Source: CAD feature listing. Evaluate the final solid. Frame: model axes, mm. A direction names the side the tool comes from. Coordinates: 2 decimals unless noted, no trailing zeros. Order: outer loops, then holes, each group sorted by start corner. A loop starts at its lowest first (then second) coordinate and runs counter-clockwise, first axis right, second up. Notation, with made-up numbers: (80.5, -24.5) - (135.5, -24.5) arc R22 cw to (135.5, -16.5) - close; hole circle Ø5 at (-3, 35). An arc over 180 degrees is marked (long way). One line per question, with ' | ' between items. Start each with the question number.
(1) Section A-A (z = 332). Return the cut outline in (x, y), then the cut area to 3 significant figures.
(2) Contact query for flat-ended pins moving along their axis: P1, Ø7.5, axis at x = 186.5, y = -11.5, coming from the +Z side; P2, Ø1, axis at x = 257, z = 582.5, coming from the +Y side; P3, Ø1, axis at x = 648.5, z = 276.5, coming from the +Y side; P4, Ø8, axis at y = 127, z = 201, coming from the -X side. Output: stop coordinate, or through.
(3) Section D-D (y = 298). Return the cut outline in (x, z).
(4) Section B-B (x = 333.5). Return the cut outline in (y, z), then the cut area to 3 significant figures.
(5) Section C-C (z = 137). Return the cut outline in (x, y).
(6) Line query: line 1 along Y through (x, z) = (148, 661); line 2 along X through (y, z) = (92.5, 163); line 3 along Z through (x, y) = (85, 84). Output: solid intervals per line, ascending.
(7) Draft query along Y for faces 1 (the cylindrical face through (396.499, 337.313, 528.478)), 2 (the cylindrical face through (540.41, 518.921, 156.835)), 3 (the cylindrical face through (231.034, 155.903, 549.168)). Return one class per face: +Y half, -Y half, draft (parallel to the pull), parting line (faces both ways), or undercut.
(8) Access query for faces 4 (the flat face through (134.52, 100.89, 183.71)), 5 (the flat face through (400.62, 376.14, 236.75)), 6 (the cylindrical face through (277.117, 188.816, 183.741)). Directions: +Z, -Z, +X, -X, +Y, -Y. A direction counts if a zero-diameter tool reaches every point of the face in a straight line with its end or side. Return the directions, or none.
from build123d import *

# Parameters (mm, degrees)
BOSS_EXTRUDE1_DEPTH  = 152.4
CUT_EXTRUDE1_DEPTH   = 406.4
BOSS_EXTRUDE2_DEPTH  = 406.4
CUT_EXTRUDE3_DEPTH   = 508
BOSS_EXTRUDE3_DEPTH  = 25.4
BOSS_EXTRUDE4_DEPTH  = 25.4
BOSS_EXTRUDE5_DEPTH  = 12.7
BOSS_EXTRUDE6_DEPTH  = 12.7
CUT_EXTRUDE4_START   = -406.4
CUT_EXTRUDE4_DEPTH   = 406.4
FILLET1_R            = 25.4
SKETCH16_W           = 406.4
SKETCH16_H           = 431.79999999999995
BOSS_EXTRUDE8_DEPTH  = 5.08
CUT_EXTRUDE5_DEPTH   = 508
SKETCH20_W           = 25.39999999999924
SKETCH20_H           = 279.40000000000003
CUT_EXTRUDE6_DEPTH   = 508
BOSS_EXTRUDE9_DEPTH  = 40.64
SKETCH22_R           = 63.50000000000003
SKETCH22_R_2         = 63.49999999999997
BOSS_EXTRUDE10_DEPTH = 40.64
SKETCH23_R           = 38.1
CUT_EXTRUDE7_DEPTH   = 279.4
SKETCH24_W           = 279.4
SKETCH24_H           = 50.542616051246114
CUT_EXTRUDE8_DEPTH   = 182.88000000000048
SKETCH25_R           = 38.1
BOSS_EXTRUDE11_DEPTH = 279.4
BOSS_EXTRUDE12_DEPTH = 63.50000000000077
BOSS_EXTRUDE14_DEPTH = 63.50000000000077
SKETCH32_W           = 67.04968691962685
SKETCH32_H           = 63.49999999999994
SKETCH32_W_2         = 67.73333333333292
SKETCH32_H_2         = 63.49999999999997
BOSS_EXTRUDE15_DEPTH = 101.6
CUT_EXTRUDE9_DEPTH   = 25.4
SKETCH34_W           = 25.40000000000001
SKETCH34_H           = 101.6
CUT_EXTRUDE11_DEPTH  = 304.8
SKETCH36_R           = 12.7
BOSS_EXTRUDE16_DEPTH = 317.5


with BuildPart() as part:
    # Sketch1 → Boss-Extrude1 (new body)
    with BuildSketch(Plane(origin=(0, 0, 0), x_dir=(1, 0, 0), z_dir=(0, 1, 0))):
        Polygon((0, 0), (812.8, 0), (812.8000000000001, -711.1999999999999), (0, -711.1999999999999), align=None)
    extrude(amount=BOSS_EXTRUDE1_DEPTH)

    # Sketch2 → Cut-Extrude1 (cut)
    with BuildSketch(Plane(origin=(0, 0, 152.4), x_dir=(-1, 0, 0), z_dir=(0, 0, -1))):
        Polygon((0, 0), (-203.2, 152.4), (0, 152.4), align=None)
    extrude(amount=-CUT_EXTRUDE1_DEPTH, mode=Mode.SUBTRACT)

    # Sketch5 → Boss-Extrude2 (add)
    with BuildSketch(Plane.XY.offset(558.8)):
        Polygon((203.2, 152.4), (521.495119519974, 548.3194575791465), (554.1241709988542, 522.0876883607381), (256.91779556245336, 152.39999999999998), align=None)
    extrude(amount=-BOSS_EXTRUDE2_DEPTH)

    # Sketch6 → Cut-Extrude3 (cut)
    with BuildSketch(Plane(origin=(472.48898283734724, 587.7174054041558, 0), x_dir=(0.7793690109825708, -0.6265651959054618, 0), z_dir=(0.6265651959054618, 0.7793690109825708, 0))):
        Polygon((62.87924717566551, -203.2), (104.74523237533951, -203.2), (104.74523237533951, -508), (62.87924717566555, -508), align=None)
    extrude(amount=-CUT_EXTRUDE3_DEPTH, mode=Mode.SUBTRACT)

    # Sketch8 → Boss-Extrude3 (add)
    with BuildSketch(Plane(origin=(81.63518816150813, -65.62971704341768, 0), x_dir=(0, 0, -1), z_dir=(0.7793690109825717, -0.6265651959054606, 0))):
        Polygon((-558.8, 754.0938850817336), (-508, 754.0938850817336), (-508, 246.0938850817336), (-558.7999999999998, 246.0938850817336), align=None)
    extrude(amount=BOSS_EXTRUDE3_DEPTH)

    # Sketch9 → Boss-Extrude4 (add)
    with BuildSketch(Plane(origin=(81.63518816150813, -65.62971704341768, 0), x_dir=(0, 0, -1), z_dir=(0.7793690109825717, -0.6265651959054606, 0))):
        Polygon((-203.2, 754.0938850817341), (-152.39999999999998, 754.0938850817341), (-152.39999999999998, 246.09388508173413), (-203.19999999999993, 246.09388508173413), align=None)
    extrude(amount=BOSS_EXTRUDE4_DEPTH)

    # Sketch10 → Boss-Extrude5 (add)
    with BuildSketch(Plane.XY.offset(203.2)):
        Polygon((203.1999999999997, 152.40000000000092), (521.4951195199743, 548.319457579147), (573.920143877812, 506.1729323847398), (289.50826251979043, 152.39999999999992), (256.9177955624533, 152.39999999999986), (235.82905147888056, 126.16823078159206), align=None)
    extrude(amount=BOSS_EXTRUDE5_DEPTH)

    # Sketch11 → Boss-Extrude6 (add)
    with BuildSketch(Plane(origin=(0, 0, 508), x_dir=(-1, 0, 0), z_dir=(0, 0, -1))):
        Polygon((-573.9201438778116, 506.1729323847395), (-289.5082625197906, 152.40000000000015), (-256.91779556245325, 152.39999999999995), (-235.82905147888056, 126.16823078159206), (-203.1999999999997, 152.40000000000092), (-521.4951195199743, 548.319457579147), align=None)
    extrude(amount=BOSS_EXTRUDE6_DEPTH)

    # Sketch12 → Cut-Extrude4 (cut)
    with BuildSketch(Plane(origin=(0, 0, 152.39999999999975), x_dir=(-1, 0, 0), z_dir=(0, 0, -1)).offset(CUT_EXTRUDE4_START)):
        Polygon((-272.8899527583018, 152.4), (-543.4408043502763, 488.93153894227703), (-512.5781156253607, 513.7432601354462), (-222.08015203498906, 152.39999999999998), align=None)
    extrude(amount=CUT_EXTRUDE4_DEPTH, mode=Mode.SUBTRACT)

    # Fillet1
    fillet1_edges = [part.edges().sort_by_distance(p)[0] for p in [
        (547.7076316988932, 527.2461949819434, 215.89999999999998),
        (547.707631698893, 527.2461949819433, 495.3),
        (547.707631698893, 527.2461949819432, 152.39999999999998),
        (521.4951195199742, 548.3194575791467, 184.14999999999998),
        (547.7076316988928, 527.246194981943, 558.8),
        (521.4951195199742, 548.3194575791467, 527.05),
        (573.9201438778116, 506.17293238473945, 527.05),
        (573.920143877812, 506.17293238473985, 184.14999999999998),
    ]]
    fillet(fillet1_edges, radius=FILLET1_R)

    # Sketch16 → Boss-Extrude8 (add)
    with BuildSketch(Plane(origin=(101.43116104046555, -81.54447301941644, 0), x_dir=(0, 0, -1), z_dir=(0.7793690109825715, -0.6265651959054606, 0))):
        with Locations((-355.59999999999997, 512.7938850817336)):
            Rectangle(SKETCH16_W, SKETCH16_H)
    extrude(amount=BOSS_EXTRUDE8_DEPTH)

    # Sketch18 → Cut-Extrude5 (cut)
    with BuildSketch(Plane(origin=(154.19386331737303, 191.79794782500986, 0), x_dir=(0.7793690109825709, -0.6265651959054616, 0), z_dir=(0.6265651959054614, 0.7793690109825708, 0))):
        Polygon((62.8792471756653, -215.89999999999998), (4.163e-14, -215.89999999999998), (4.163e-14, -495.3), (62.8792471756653, -495.3), (104.74523237533926, -495.3), (130.1452323753393, -495.3), (130.14523237533894, -215.89999999999998), (104.74523237533926, -215.89999999999998), align=None)
    extrude(amount=-CUT_EXTRUDE5_DEPTH, mode=Mode.SUBTRACT)

    # Sketch20 → Cut-Extrude6 (cut)
    with BuildSketch(Plane(origin=(154.19386331737306, 191.79794782500986, 0), x_dir=(-0.7793690109825709, 0.6265651959054614, 0), z_dir=(-0.6265651959054614, -0.7793690109825709, 0))):
        with Locations((-117.44523237533932, -355.6)):
            Rectangle(SKETCH20_W, SKETCH20_H)
    extrude(amount=-CUT_EXTRUDE6_DEPTH, mode=Mode.SUBTRACT)

    # Sketch21 → Boss-Extrude9 (add)
    with BuildSketch(Plane(origin=(91.33693287972456, -73.42932864502501, 0), x_dir=(0, 0, 1), z_dir=(-0.7793690109825776, 0.6265651959054531, 0))):
        with BuildLine():
            Line((209.39759999999998, 562.2934659364746), (289.1018868532613, 546.366600042237))
            Line((289.1018868532613, 546.366600042237), (210.56545348218663, 525.4269956202154))
            ThreePointArc((210.56545348218663, 525.4269956202154), (185.1552700280405, 511.30785991563), (158.90239999999997, 523.7904170057728))
            Line((158.90239999999997, 523.7904170057728), (79.93520930816898, 543.0419414711238))
            Line((79.93520930816898, 543.0419414711238), (158.90239999999997, 562.2934659364746))
            ThreePointArc((158.90239999999997, 562.2934659364746), (184.14999999999998, 574.7919414711238), (209.39759999999998, 562.2934659364746))
        make_face()
        with BuildLine():
            Line((289.1018868532613, 292.366600042237), (210.56545348218663, 271.42699562021545))
            ThreePointArc((210.56545348218663, 271.42699562021545), (185.15527002804046, 257.30785991563005), (158.90239999999997, 269.7904170057729))
            Line((158.90239999999997, 269.7904170057729), (79.93520930816898, 289.0419414711237))
            Line((79.93520930816898, 289.0419414711237), (158.90239999999997, 308.29346593647455))
            ThreePointArc((158.90239999999997, 308.29346593647455), (184.14999999999998, 320.7919414711238), (209.39759999999998, 308.29346593647455))
            Line((209.39759999999998, 308.29346593647455), (289.1018868532613, 292.366600042237))
        make_face()
        with BuildLine():
            Line((632.0018868532613, 292.36660004223734), (553.4654534821866, 271.4269956202158))
            ThreePointArc((553.4654534821866, 271.4269956202158), (528.0552700280405, 257.3078599156303), (501.8024, 269.79041700577324))
            Line((501.8024, 269.79041700577324), (422.835209308169, 289.04194147112406))
            Line((422.835209308169, 289.04194147112406), (501.8024, 308.2934659364749))
            ThreePointArc((501.8024, 308.2934659364749), (527.0500000000001, 320.791941471124), (552.2976, 308.2934659364749))
            Line((552.2976, 308.2934659364749), (632.0018868532613, 292.36660004223734))
        make_face()
        with BuildLine():
            Line((501.8024, 523.7904170057732), (422.835209308169, 543.041941471124))
            Line((422.835209308169, 543.041941471124), (501.8024, 562.293465936475))
            ThreePointArc((501.8024, 562.293465936475), (527.0500000000001, 574.791941471124), (552.2976, 562.293465936475))
            Line((552.2976, 562.293465936475), (632.0018868532613, 546.3666000422373))
            Line((632.0018868532613, 546.3666000422373), (553.4654534821866, 525.4269956202157))
            ThreePointArc((553.4654534821866, 525.4269956202157), (528.0552700280405, 511.3078599156302), (501.8024, 523.7904170057732))
        make_face()
    extrude(amount=BOSS_EXTRUDE9_DEPTH)

    # Sketch22 → Boss-Extrude10 (add)
    with BuildSketch(Plane(origin=(91.33693287972456, -73.42932864502501, 0), x_dir=(0, 0, 1), z_dir=(-0.7793690109825776, 0.6265651959054531, 0))):
        with Locations((184.14999999999998, 670.4976110611291)):
            Circle(SKETCH22_R)
        with Locations((519.43, 670.4976110611292)):
            Circle(SKETCH22_R_2)
    extrude(amount=BOSS_EXTRUDE10_DEPTH)

    # Sketch23 → Cut-Extrude7 (cut)
    with BuildSketch(Plane.XY.offset(215.89999999999998)):
        with Locations((203.2, 12.700000000001378)):
            Circle(SKETCH23_R)
    extrude(amount=CUT_EXTRUDE7_DEPTH, mode=Mode.SUBTRACT)

    # Sketch24 → Cut-Extrude8 (cut)
    with BuildSketch(Plane.ZY):
        with Locations((355.59999999999997, 25.271308025623057)):
            Rectangle(SKETCH24_W, SKETCH24_H)
    extrude(amount=-CUT_EXTRUDE8_DEPTH, mode=Mode.SUBTRACT)

    # Sketch25 → Boss-Extrude11 (add)
    with BuildSketch(Plane.XY.offset(215.89999999999998)):
        with Locations((203.2, 12.700000000001378)):
            Circle(SKETCH25_R)
    extrude(amount=BOSS_EXTRUDE11_DEPTH)

    # Sketch26 → Boss-Extrude12 (add)
    with BuildSketch(Plane.XY.offset(215.89999999999998)):
        Polygon((0, 0), (-6.22e-15, 50.8), (67.73333333333265, 50.8), align=None)
    extrude(amount=-BOSS_EXTRUDE12_DEPTH)

    # Sketch30 → Boss-Extrude14 (add)
    with BuildSketch(Plane(origin=(0, 0, 495.3), x_dir=(-1, 0, 0), z_dir=(0, 0, -1))):
        Polygon((2.776e-14, -2.776e-14), (0, 50.79999999999997), (-67.73333333333278, 50.79999999999996), align=None)
    extrude(amount=-BOSS_EXTRUDE14_DEPTH)

    # Sketch32 → Boss-Extrude15 (add)
    with BuildSketch(Plane(origin=(5.2e-15, 50.79999999999997, 0), x_dir=(1, -1e-16, 0), z_dir=(1e-16, 1, 0))):
        with Locations((33.524843459813425, -527.05)):
            Rectangle(SKETCH32_W, SKETCH32_H)
        with Locations((33.86666666666645, -184.14999999999998)):
            Rectangle(SKETCH32_W_2, SKETCH32_H_2)
    extrude(amount=BOSS_EXTRUDE15_DEPTH)

    # Sketch33 → Cut-Extrude9 (cut)
    with BuildSketch(Plane.XY.offset(215.89999999999998)):
        Polygon((12.69999999999997, 134.2251095976107), (38.099999999999966, 134.2251095976107), (38.09999999999998, 32.625109597610695), (12.699999999999983, 32.625109597610695), align=None)
    extrude(amount=-CUT_EXTRUDE9_DEPTH, mode=Mode.SUBTRACT)

    # Sketch34 → Cut-Extrude11 (cut)
    with BuildSketch(Plane.XY.offset(215.89999999999998)):
        with Locations((25.399999999999977, 83.4251095976107)):
            Rectangle(SKETCH34_W, SKETCH34_H)
    extrude(amount=CUT_EXTRUDE11_DEPTH, mode=Mode.SUBTRACT)

    # Sketch36 → Boss-Extrude16 (add)
    with BuildSketch(Plane.XY.offset(190.49999999999997)):
        with Locations(Location((29.63333333333292, 108.82510959761069, 0), (0, 0, 311.810314896))):
            Circle(SKETCH36_R)
    extrude(amount=BOSS_EXTRUDE16_DEPTH)


solid = part.part
Response values:
1) outline: circle Ø25.4 at (29.63, 108.83); (207.62, 50.54) arc R38.1 ccw (long way) to (239.12, 0) - (812.8, 0) - (812.8, 152.4) - (296.03, 152.4) - (561.96, 483.19) - (558.01, 486.38) - close | area: 93,900 mm²
2) P1: stops at z = 495.3 | P2: stops at y = 181.63 | P3: stops at y = 152.4 | P4: stops at x = 0
3) outline: (320.25, 152.4) - (339.13, 152.4) - (339.13, 215.9) - (320.25, 215.9) - close; (320.25, 495.3) - (339.13, 495.3) - (339.13, 558.8) - (320.25, 558.8) - close; (389.94, 152.4) - (413.08, 152.4) - (413.08, 558.8) - (389.94, 558.8) - (389.94, 495.3) - (406.56, 495.3) - (406.56, 215.9) - (389.94, 215.9) - close
4) outline: (0, 0) - (152.4, 0) - (152.4, 711.2) - (0, 711.2) - close; (199.01, 152.4) - (227.79, 152.4) - (227.79, 215.9) - (207.12, 215.9) - (207.12, 495.3) - (227.79, 495.3) - (227.79, 558.8) - (199.01, 558.8) - close; (290.99, 152.4) - (314.48, 152.4) - (314.48, 215.9) - (290.99, 215.9) - close; (290.99, 495.3) - (314.48, 495.3) - (314.48, 558.8) - (290.99, 558.8) - close | area: 117,000 mm²
5) outline: (0, 0) - (812.8, 0) - (812.8, 152.4) - (272.89, 152.4) - (281.16, 162.68) - (249.48, 188.15) - (232.05, 166.46) - (249.54, 152.4) - (0, 152.4) - close; (391.2, 364.42) - (422.87, 338.96) - (440.3, 360.64) - (408.63, 386.11) - close; (453.12, 441.45) - (484.8, 415.99) - (538.1, 482.29) - (506.42, 507.75) - close
6) line 1: y = 0 to 152.4 | line 2: x = 0 to 67.73, 123.33 to 812.8 | line 3: z = 0 to 152.4, 558.8 to 711.2
7) face 1: undercut | face 2: +Y half | face 3: undercut
8) face 4: +Y | face 5: -X, +Y | face 6: none
